Read the model definition and answer for the solid it produces. Units are mm, in the model's axes. Face numbers are marked on the shaded views. Give positions to 0.01 mm unless a question says otherwise; leave off trailing zeros. Order: outer loops, then holes, each group sorted by start corner. A loop starts at its lowest first (then second) coordinate and runs counter-clockwise, first axis right, second up. Notation, with made-up numbers: (-39.5, 42) - (-12.5, 42) arc R23 ccw to (-12.5, 78) - close; hole circle Ø5 at (11, 22). An arc over 180 degrees is marked (long way). Write each question's results on one line, items separated by ' | '. Start each with the question number.
Q1. Flat-ended cylindrical pins translate along their axes: P1, Ø6, axis at x = 3.5, y = 17, coming from the +Z side; P2, Ø13, axis at x = 34.5, y = 11.5, coming from the -Z side; P3, Ø5.5, axis at x = 8.5, y = -5, coming from the -Z side; P4, Ø2, axis at x = 42.5, z = 3, coming from the -Y side. Find the tip coordinate at first contact, or state that the pin passes through.
Q2. Find section D-D on x = 6.5. Give the vertices of the cut face in (y, z).
Q3. For a pull along X with two mould halves and no side action, classify the marked faces 1 and 2 as +X half, -X half, draft (parallel to the pull), parting line (faces both ways), or undercut.
Q4. Find section B-B on z = 2.6. Give the vertices of the cut face in (x, y).
Q5. Find section C-C on y = -1. Give the vertices of the cut face in (x, z).
Q6. Find section A-A on x = -30. Give the vertices of the cut face in (y, z), and give its area (3 significant figures).
Q7. Find the intervals of material crossed by line 1 along Y through (x, z) = (-30, 2.2); line 2 along X through (y, z) = (-16, 3.7); line 3 along X through (y, z) = (1, 3.3), in increasing order. Write a range as from..to.
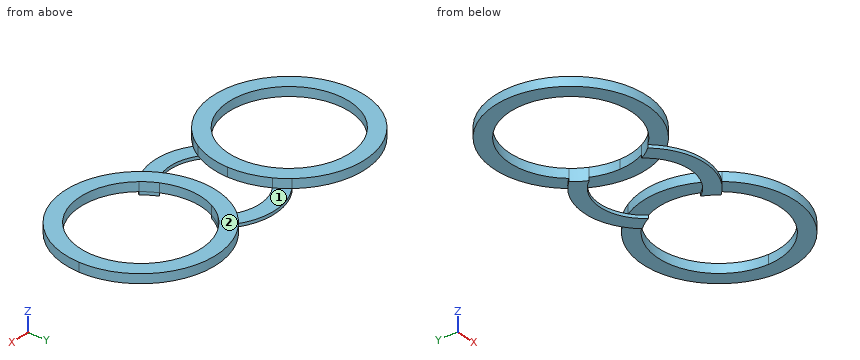
from build123d import *

# Parameters (mm, degrees)
F0_R     = 19.75
F0_R_2   = 14.75
F1_DEPTH = 1
F3_DEPTH = 3
F4_DEPTH = 25


with BuildPart() as f1:
    # F0 (on Top) → F1 (new body)
    with BuildSketch(Plane.XY):
        Circle(F0_R)
        Circle(F0_R_2, mode=Mode.SUBTRACT)
    extrude(amount=F1_DEPTH)

    # F2 (on face) → F3 (join)
    with BuildSketch(Plane.XY.offset(1)):
        with BuildLine():
            ThreePointArc((-14.834375, -13.038551237), (-50, 0), (-14.834375, 13.038551237))
            ThreePointArc((-14.834375, 13.038551237), (-13.0644777856, 14.8115468533), (-11.084375, 16.346226808))
            ThreePointArc((-11.084375, 16.346226808), (-55, 0), (-11.084375, -16.346226808))
            ThreePointArc((-11.084375, -16.346226808), (-13.0644777856, -14.8115468533), (-14.834375, -13.038551237))
        make_face()
        with BuildLine():
            ThreePointArc((-11.959375, 8.6334147132), (-10.4959940012, 4.4264828024), (-10, 0))
            ThreePointArc((-10, 0), (-10.4959940012, -4.4264828024), (-11.959375, -8.6334147132))
            ThreePointArc((-11.959375, -8.6334147132), (-10.2456029754, -10.6108491493), (-8.209375, -12.2543323812))
            ThreePointArc((-8.209375, -12.2543323812), (-5.8156494298, -6.3338130301), (-5, 0))
            ThreePointArc((-5, 0), (-5.8156494298, 6.3338130301), (-8.209375, 12.2543323812))
            ThreePointArc((-8.209375, 12.2543323812), (-10.2456029754, 10.6108491493), (-11.959375, 8.6334147132))
        make_face()
        with BuildLine():
            ThreePointArc((-14.834375, 13.038551237), (-13.2514159788, 10.9309163974), (-11.959375, 8.6334147132))
            ThreePointArc((-11.959375, 8.6334147132), (-10.2456029754, 10.6108491493), (-8.209375, 12.2543323812))
            ThreePointArc((-8.209375, 12.2543323812), (-9.5443015943, 14.3723485462), (-11.084375, 16.346226808))
            ThreePointArc((-11.084375, 16.346226808), (-13.0644777856, 14.8115468533), (-14.834375, 13.038551237))
        make_face()
        with BuildLine():
            ThreePointArc((-8.209375, -12.2543323812), (-10.2456029754, -10.6108491493), (-11.959375, -8.6334147132))
            ThreePointArc((-11.959375, -8.6334147132), (-13.2514159788, -10.9309163974), (-14.834375, -13.038551237))
            ThreePointArc((-14.834375, -13.038551237), (-13.0644777856, -14.8115468533), (-11.084375, -16.346226808))
            ThreePointArc((-11.084375, -16.346226808), (-9.5443015943, -14.3723485462), (-8.209375, -12.2543323812))
        make_face()
        with BuildLine():
            ThreePointArc((55, 0), (38.7209338663, 23.4295819958), (11.084375, 16.346226808))
            ThreePointArc((11.084375, 16.346226808), (13.0644777856, 14.8115468533), (14.834375, 13.038551237))
            ThreePointArc((14.834375, 13.038551237), (36.9529669926, 18.7524998334), (50, 0))
            ThreePointArc((50, 0), (36.9529669926, -18.7524998334), (14.834375, -13.038551237))
            ThreePointArc((14.834375, -13.038551237), (13.0644777856, -14.8115468533), (11.084375, -16.346226808))
            ThreePointArc((11.084375, -16.346226808), (38.7209338663, -23.4295819958), (55, 0))
        make_face()
        with BuildLine():
            ThreePointArc((11.959375, -8.6334147132), (10.2456029754, -10.6108491493), (8.209375, -12.2543323812))
            ThreePointArc((8.209375, -12.2543323812), (9.5443015943, -14.3723485462), (11.084375, -16.346226808))
            ThreePointArc((11.084375, -16.346226808), (13.0644777856, -14.8115468533), (14.834375, -13.038551237))
            ThreePointArc((14.834375, -13.038551237), (13.2514159788, -10.9309163974), (11.959375, -8.6334147132))
        make_face()
        with BuildLine():
            ThreePointArc((11.959375, 8.6334147132), (10.2456029754, 10.6108491493), (8.209375, 12.2543323812))
            ThreePointArc((8.209375, 12.2543323812), (5, 0), (8.209375, -12.2543323812))
            ThreePointArc((8.209375, -12.2543323812), (10.2456029754, -10.6108491493), (11.959375, -8.6334147132))
            ThreePointArc((11.959375, -8.6334147132), (10, 0), (11.959375, 8.6334147132))
        make_face()
        with BuildLine():
            ThreePointArc((11.084375, 16.346226808), (9.5443015943, 14.3723485462), (8.209375, 12.2543323812))
            ThreePointArc((8.209375, 12.2543323812), (10.2456029754, 10.6108491493), (11.959375, 8.6334147132))
            ThreePointArc((11.959375, 8.6334147132), (13.2514159788, 10.9309163974), (14.834375, 13.038551237))
            ThreePointArc((14.834375, 13.038551237), (13.0644777856, 14.8115468533), (11.084375, 16.346226808))
        make_face()
    extrude(amount=F3_DEPTH)

    # F4 (cut): faces of the model
    f4_faces = [f1.faces().sort_by_distance(p)[0] for p in [
        (16.0717214062, 0, 1),
        (-16.0717214062, 0, 1),
    ]]
    extrude(f4_faces, amount=-F4_DEPTH, mode=Mode.SUBTRACT)


solid = f1.part
Working result:
1) P1: z = 1 | P2: through | P3: z = 1 | P4: y = -22.2
2) outline: (-18.65, 0) - (-13.24, 0) - (-13.24, 1) - (-18.65, 1) - close; (-8.53, 1) - (8.53, 1) - (8.53, 4) - (-8.53, 4) - close; (13.24, 0) - (18.65, 0) - (18.65, 1) - (13.24, 1) - close
3) face 1: undercut | face 2: draft
4) outline: circle Ø50 at (-30, 0); circle Ø50 at (30, 0); hole circle Ø40 at (-30, 0); hole circle Ø40 at (30, 0)
5) outline: (-54.98, 1) - (-49.97, 1) - (-49.97, 4) - (-54.98, 4) - close; (-10.03, 1) - (-5.02, 1) - (-5.02, 4) - (-10.03, 4) - close; (5.02, 1) - (10.03, 1) - (10.03, 4) - (5.02, 4) - close; (49.97, 1) - (54.98, 1) - (54.98, 4) - (49.97, 4) - close
6) outline: (-25, 1) - (-20, 1) - (-20, 4) - (-25, 4) - close; (20, 1) - (25, 1) - (25, 4) - (20, 4) - close | area: 30.0 mm²
7) line 1: -25..-20, 20..25 | line 2: -49.21..-42, -18..-10.79, 10.79..18, 42..49.21 | line 3: -54.98..-49.97, -10.03..-5.02, 5.02..10.03, 49.97..54.98
